Check sheet for the drawn part. Datum: minimum x, y, z corner. Units: mm. Coordinates: 2 decimals unless noted, no trailing zeros. Loops run counter-clockwise (first coordinate to the right, second up) from the corner with the lowest first, then second, coordinate; pieces in that order, holes last. Notation, with made-up numbers: (49.5, 33.25) -> (86.5, 33.25) arc R36 cw to (86.5, 71.25) -> close; hole circle Ø1 at (-38.75, 10.25). An arc over 180 degrees is marked (long way). Use CSV: the item, a comma, the result in double quotes. Start each with the question number.
1. Sectioned sample at B-B, the plane x = 75. Record the cut outline in (y, z), and give its area (3 significant figures).
2. Thickness scan on L1, parallel to Y at x = 111, z = 1.45; L2, parallel to Y at x = 75, z = 0.9. Record the ranges inside material, lowest first.
3. Sectioned sample at C-C, the plane x = 118. Record the cut outline in (y, z).
4. Sectioned sample at D-D, the plane z = 2.45. Count the separate pieces of the cut face and the enclosed holes in it, and give its area (3 significant figures).
5. Sectioned sample at A-A, the plane y = 23.15. Record the cut outline in (x, z), and give its area (3 significant figures).
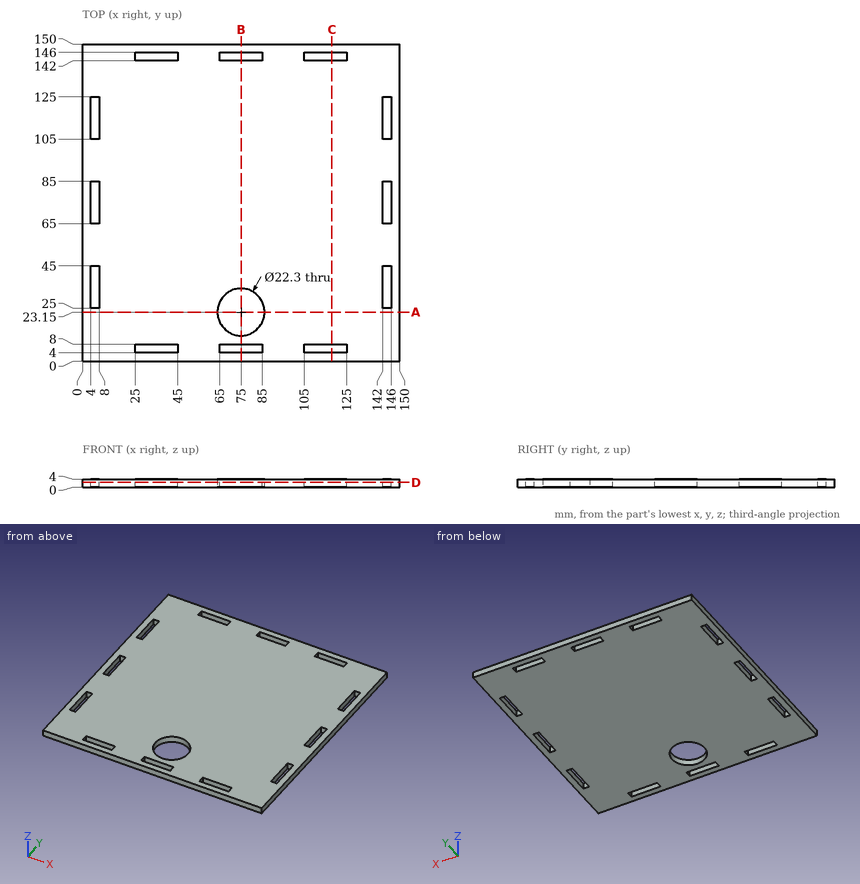
Completed:
1,outline,"(0, 0) -> (4, 0) -> (4, 4) -> (0, 4) -> close; (8, 0) -> (12, 0) -> (12, 4) -> (8, 4) -> close; (34.3, 0) -> (142, 0) -> (142, 4) -> (34.3, 4) -> close; (146, 0) -> (150, 0) -> (150, 4) -> (146, 4) -> close"
1,area,"479 mm²"
2,L1,"0 to 4, 8 to 142, 146 to 150"
2,L2,"0 to 4, 8 to 12, 34.3 to 142, 146 to 150"
3,outline,"(0, 0) -> (4, 0) -> (4, 4) -> (0, 4) -> close; (8, 0) -> (142, 0) -> (142, 4) -> (8, 4) -> close; (146, 0) -> (150, 0) -> (150, 4) -> (146, 4) -> close"
4,separate pieces,"1"
4,enclosed holes,"13"
4,area,"21,100 mm²"
5,outline,"(0, 0) -> (63.85, 0) -> (63.85, 4) -> (0, 4) -> close; (86.15, 0) -> (150, 0) -> (150, 4) -> (86.15, 4) -> close"
5,area,"511 mm²"
